```python
from build123d import *

# Parameters (mm, degrees)
F0_R     = 6.35
F1_DEPTH = 12.7
F3_R     = 2.54
F3_R_2   = 7.62
F5_DEPTH = 89.8035612107


with BuildPart() as f1:
    # F0 (on Top) → F1 (new body)
    with BuildSketch(Plane.XY):
        with BuildLine():
            Line((-31.75, -19.05), (0, -19.05))
            Line((0, -19.05), (0, 19.05))
            Line((0, 19.05), (-31.75, 19.05))
            Line((-31.75, 19.05), (-31.75, 31.75))
            ThreePointArc((-31.75, 31.75), (-44.45, 44.45), (-57.15, 31.75))
            Line((-57.15, 31.75), (-57.15, 6.35))
            Line((-57.15, 6.35), (-44.45, 6.35))
            ThreePointArc((-44.45, 6.35), (-38.1, 0), (-44.45, -6.35))
            Line((-44.45, -6.35), (-57.15, -6.35))
            Line((-57.15, -6.35), (-57.15, -31.75))
            ThreePointArc((-57.15, -31.75), (-44.45, -44.45), (-31.75, -31.75))
            Line((-31.75, -31.75), (-31.75, -19.05))
        make_face()
        with Locations((-44.45, -31.75)):
            Circle(F0_R, mode=Mode.SUBTRACT)
        with Locations((-44.45, 31.75)):
            Circle(F0_R, mode=Mode.SUBTRACT)
        with BuildLine():
            Line((0, 19.05), (0, -19.05))
            Line((0, -19.05), (31.75, -19.05))
            Line((31.75, -19.05), (31.75, -31.75))
            ThreePointArc((31.75, -31.75), (44.45, -44.45), (57.15, -31.75))
            Line((57.15, -31.75), (57.15, 31.75))
            ThreePointArc((57.15, 31.75), (44.45, 44.45), (31.75, 31.75))
            Line((31.75, 31.75), (31.75, 19.05))
            Line((31.75, 19.05), (0, 19.05))
        make_face()
        with Locations((44.45, -31.75)):
            Circle(F0_R, mode=Mode.SUBTRACT)
        with Locations((44.45, 31.75)):
            Circle(F0_R, mode=Mode.SUBTRACT)
    extrude(amount=-F1_DEPTH)

    # F3 (on face) → F4 (join, up to the next surface of F1)
    with BuildSketch(Plane(origin=(28.575, 0, 28.575), x_dir=(0, 1, 0), z_dir=(0.7071067812, 0, 0.7071067812))):
        with BuildLine():
            Line((-19.05, -40.4111525448), (0, -40.4111525448))
            Line((0, -40.4111525448), (19.05, -40.4111525448))
            Line((19.05, -40.4111525448), (19.05, -5.4861525448))
            ThreePointArc((19.05, -5.4861525448), (0, 13.5638474552), (-19.05, -5.4861525448))
            Line((-19.05, -5.4861525448), (-19.05, -40.4111525448))
        make_face()
        with Locations((-7.4648727041, -15.7606683734)):
            Circle(F3_R, mode=Mode.SUBTRACT)
        with Locations((7.4648727041, -15.7606683734)):
            Circle(F3_R, mode=Mode.SUBTRACT)
        with Locations((-12.0784177569, -1.5616367162)):
            Circle(F3_R, mode=Mode.SUBTRACT)
        with Locations((0, -5.4861525448)):
            Circle(F3_R_2, mode=Mode.SUBTRACT)
        with Locations((12.0784177569, -1.5616367162)):
            Circle(F3_R, mode=Mode.SUBTRACT)
        with Locations((0, 7.2138474552)):
            Circle(F3_R, mode=Mode.SUBTRACT)
    extrude(until=Until.NEXT, dir=(-0.7071067812, 0, -0.7071067812))

    # F3 (on face) → F5 (cut, through all)
    with BuildSketch(Plane(origin=(28.575, 0, 28.575), x_dir=(0, 1, 0), z_dir=(0.7071067812, 0, 0.7071067812))):
        with Locations((0, 7.2138474552)):
            Circle(F3_R)
        with Locations((12.0784177569, -1.5616367162)):
            Circle(F3_R)
        with Locations((7.4648727041, -15.7606683734)):
            Circle(F3_R)
        with Locations((-7.4648727041, -15.7606683734)):
            Circle(F3_R)
        with Locations((-12.0784177569, -1.5616367162)):
            Circle(F3_R)
        with Locations((0, -5.4861525448)):
            Circle(F3_R_2)
    extrude(amount=-F5_DEPTH, mode=Mode.SUBTRACT)


solid = f1.part
```
Input: part model. Units: mm. Frame: model coordinates. A direction names the side the tool comes from. Coordinates: 2 decimals unless noted, no trailing zeros. Order: outer loops, then holes, each group sorted by start corner. A loop starts at its lowest first (then second) coordinate and runs counter-clockwise, first axis right, second up. Notation, with made-up numbers: (26.5, 30) - (59.5, 30) arc R13 ccw to (59.5, 42) - close; hole circle Ø1 at (37.25, 51). An arc over 180 degrees is marked (long way). Put each result on its own line as item: value.
1. Cut plane D-D on z = 20.5. State how many separate pieces and enclosed holes the cut face has, then the cut area to 3 significant figures.
Report:
separate pieces: 1
enclosed holes: 3
area: 797 mm2
2. Cut plane B-B on y = 0. Return the cut outline in (x, z), then the cut area to 3 significant figures.
Report:
outline: (-38.1, -12.7) - (-26.49, -12.7) - (21.68, 35.47) - (18.98, 38.17) - (-19.18, 0) - (-38.1, 0) - close; (-19.31, -12.7) - (-15.72, -12.7) - (27.07, 30.08) - (25.27, 31.88) - close; (5.83, -12.7) - (57.15, -12.7) - (57.15, 0) - (37.84, 19.31) - close
area: 1,530 mm2
3. Cut plane C-C on y = 30. Return the cut outline in (x, z), then the cut area to 3 significant figures.
Report:
outline: (-57.15, -12.7) - (-50.55, -12.7) - (-50.55, 0) - (-57.15, 0) - close; (-38.35, -12.7) - (-31.75, -12.7) - (-31.75, 0) - (-38.35, 0) - close; (31.75, -12.7) - (38.35, -12.7) - (38.35, 0) - (31.75, 0) - close; (50.55, -12.7) - (57.15, -12.7) - (57.15, 0) - (50.55, 0) - close
area: 335 mm2
4. Reachability of faces 4 (the face through (41, -26, 0)), 5 (the face through (44, 23, 0)), 6 (the face through (15, 19.05, -1)), 7 (the face through (31.75, -25, -6)) from +Z, -Z, +X, -X, +Y, -Y: full face, straight path, thin tool, end or side. Return the list, or none.
Report:
face 4: +Z, +X, -X, -Y
face 5: +Z, +X, -X, +Y
face 6: +Z, +Y
face 7: +Z, -Z, -Y
5. Cut plane A-A on x = 44.45. Return the cut outline in (y, z).
Report:
outline: (-44.45, -12.7) - (-38.1, -12.7) - (-38.1, 0) - (-44.45, 0) - close; (-25.4, -12.7) - (25.4, -12.7) - (25.4, 0) - (19.05, 0) - (19.05, 12.7) - (-19.05, 12.7) - (-19.05, 0) - (-25.4, 0) - close; (38.1, -12.7) - (44.45, -12.7) - (44.45, 0) - (38.1, 0) - close
6. Line query: line 1 along Y through (x, z) = (44.45, -4); line 2 along Y through (x, z) = (-44.45, -4.5); line 3 along X through (y, z) = (-21, -3). Output: solid intervals per line, ascending.
Report:
line 1: y = -44.45 to -38.1, -25.4 to 25.4, 38.1 to 44.45
line 2: y = -44.45 to -38.1, -25.4 to -6.35, 6.35 to 25.4, 38.1 to 44.45
line 3: x = -57.15 to -31.75, 31.75 to 57.15
7. Draft query along Z for faces 1 (the face through (31.75, 25, -6)), 2 (the face through (22.2, 7.13, 3.47)), 3 (the face through (-32, 1, 0)). Return one class per face: pulls with the +Z half, pulls with the -Z half, needs draft (parallel to the pull), parting line crosses it, or undercut.
Report:
face 1: needs draft
face 2: undercut
face 3: pulls with the +Z half
8. Contact query for flat-ended pins moving along their axis: pin 1 Ø6 at (x, y) = (32, -2) entering from +Z; pin 2 Ø2 at (y, z) = (6, 29.5) entering from -X; pin 3 Ø12 at (y, z) = (-7, 1.5) entering from +X; pin 4 Ø14.5 at (x, y) = (-44.45, 31.75) entering from +Z. Output: stop coordinate, or through.
Report:
pin 1: stops at z = 17.31
pin 2: stops at x = 10.59
pin 3: stops at x = 57.15
pin 4: stops at z = 0
